Verification items for the finished model (mm, model axes). Face numbers are marked on the shaded views. A direction names the side the tool comes from. Give positions to 0.01 mm unless a question says otherwise; leave off trailing zeros. Loops run counter-clockwise (first coordinate to the right, second up) from the corner with the lowest first, then second, coordinate; pieces in that order, holes last. Notation, with made-up numbers: M 30.25,55 L 71.25,55 A37 cw 71.25,93 Z; hole C 75.25,40 d9. An arc over 180 degrees is marked long. Use a Markdown table: item, result.
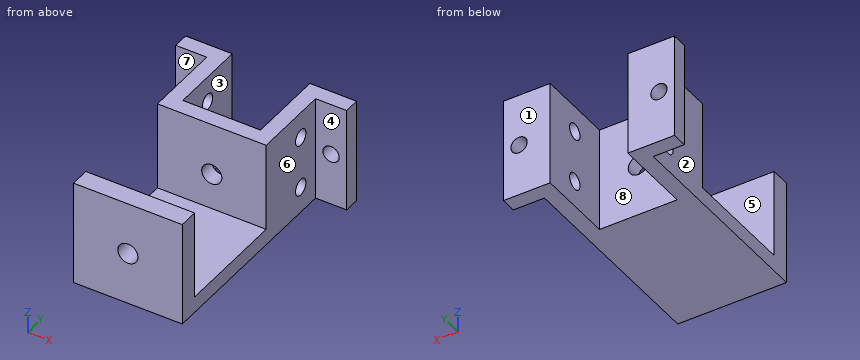
from build123d import *

# Parameters (mm, degrees)
BOSS_EXTRUDE1_DEPTH = 27
SKETCH2_R           = 2.1
CUT_EXTRUDE1_DEPTH  = 52
SKETCH3_R           = 2.1
CUT_EXTRUDE2_DEPTH  = 41.162171256
SKETCH5_W           = 28
SKETCH5_H           = 4.176671075
BOSS_EXTRUDE2_DEPTH = 34
SKETCH6_W           = 28
SKETCH6_H           = 5
BOSS_EXTRUDE3_DEPTH = 22.823328925
SKETCH7_R           = 2.6
CUT_EXTRUDE3_DEPTH  = 68.653529103


with BuildPart() as part:
    # Sketch1 → Boss-Extrude1 (new body)
    with BuildSketch(Plane.XY):
        Polygon((-14, 0), (14, 0), (14, 20), (22, 20), (22, 24), (10, 24), (10, 4), (-10, 4), (-10, 24), (-22, 24), (-22, 20), (-14, 20), align=None)
    extrude(amount=BOSS_EXTRUDE1_DEPTH)

    # Sketch2 → Cut-Extrude1 (cut, through all)
    with BuildSketch(Plane.ZY.offset(14)):
        with Locations(Location((6.75, 14, 0), (0, 0, 270))):
            Circle(SKETCH2_R)
        with Locations(Location((20.25, 14, 0), (0, 0, 270))):
            Circle(SKETCH2_R)
    extrude(amount=-CUT_EXTRUDE1_DEPTH, mode=Mode.SUBTRACT)

    # Sketch3 → Cut-Extrude2 (cut, through all)
    with BuildSketch(Plane.XZ.offset(-20)):
        with Locations(Location((-18, 13.5, 0), (0, 0, 270))):
            Circle(SKETCH3_R)
        with Locations(Location((18, 13.5, 0), (0, 0, 270))):
            Circle(SKETCH3_R)
    extrude(amount=-CUT_EXTRUDE2_DEPTH, mode=Mode.SUBTRACT)

    # Sketch5 → Boss-Extrude2 (add)
    with BuildSketch(Plane.XZ):
        with Locations((0, 2.088335538)):
            Rectangle(SKETCH5_W, SKETCH5_H)
    extrude(amount=BOSS_EXTRUDE2_DEPTH)

    # Sketch6 → Boss-Extrude3 (add)
    with BuildSketch(Plane.XY.offset(4.176671075)):
        with Locations((0, -31.5)):
            Rectangle(SKETCH6_W, SKETCH6_H)
    extrude(amount=BOSS_EXTRUDE3_DEPTH)

    # Sketch7 → Cut-Extrude3 (cut, through all)
    with BuildSketch(Plane.XZ.offset(34)):
        with Locations(Location((0, 13.5, 0), (0, 0, 270))):
            Circle(SKETCH7_R)
    extrude(amount=-CUT_EXTRUDE3_DEPTH, mode=Mode.SUBTRACT)


solid = part.part
(1) Draft check along X on the marked faces 6, 7 and 8. Enter one of: +X half, -X half, draft (parallel to the pull), parting line (faces both ways), or undercut.
Results below:
| item | result |
|---|---|
| face 6 | +X half |
| face 7 | draft |
| face 8 | undercut |
(2) Cross-section at B-B on y = 10. Record the cut outline in (x, z), then the cut area to 3 significant figures.
Results below:
| item | result |
|---|---|
| outline | M -14,0 L -10,0 L -10,27 L -14,27 Z; M 10,0 L 14,0 L 14,27 L 10,27 Z |
| area | 216 mm^2 |
(3) Set-up check for the marked faces 1, 2, 3, 4 and 5: record each of +Z, -Z, +X, -X, +Y, -Y from which the full face is reachable in a straight line by a thin tool's end or side.
Results below:
| item | result |
|---|---|
| face 1 | +Z, -Z, +X, -X, +Y |
| face 2 | +Z, -Z, -X, -Y |
| face 3 | +Z, -Z, +Y |
| face 4 | +Z, -Z, +X, -Y |
| face 5 | +Z, +X, -X |
(4) Cross-section at D-D on z = 13.5. State how many separate pieces and enclosed holes the cut face has, then the cut area to 3 significant figures.
Results below:
| item | result |
|---|---|
| separate pieces | 6 |
| enclosed holes | 0 |
| area | 396 mm^2 |
(5) Material ranges on line 1 (Z direction, x = 11.3, y = 14); line 2 (X direction, y = 22.65, z = 13.5); line 3 (Y direction, x = -1, z = 21.25), recorded low to high.
Results below:
| item | result |
|---|---|
| line 1 | 0 to 4.65, 8.85 to 18.15, 22.35 to 27 |
| line 2 | -22 to -20.1, -15.9 to -10, 10 to 15.9, 20.1 to 22 |
| line 3 | -34 to -29, 0 to 4 |
(6) Cross-section at A-A on x = -18. Record the cut outline in (y, z), then the cut area to 3 significant figures.
Results below:
| item | result |
|---|---|
| outline | M 20,0 L 24,0 L 24,11.4 L 20,11.4 Z; M 20,15.6 L 24,15.6 L 24,27 L 20,27 Z |
| area | 91.2 mm^2 |
(7) Gauge pin test, flat ends, axial feed: P1, Ø4, axis at x = 0, z = 13.5, coming from the -Y side; P2, Ø6, axis at x = 0, z = 13.5, coming from the +Y side; P3, Ø9, axis at x = -19.5, z = 15, coming from the -Y side; P4, Ø5, axis at y = 14, z = 6.75, coming from the -X side. Record the tip position at first contact, or that the pin passes through.
Results below:
| item | result |
|---|---|
| P1 | through |
| P2 | y = 4 |
| P3 | y = 20 |
| P4 | x = -14 |
(8) Cross-section at C-C on z = 24. Record the cut outline in (x, y).
Results below:
| item | result |
|---|---|
| outline | M -22,20 L -14,20 L -14,0 L 14,0 L 14,20 L 22,20 L 22,24 L 10,24 L 10,4 L -10,4 L -10,24 L -22,24 Z; M -14,-34 L 14,-34 L 14,-29 L -14,-29 Z |
